Geometry check sheet. Reference: drawing and pictorial views, mm from the part's lowest x, y, z. Give positions to 0.01 mm unless a question says otherwise; leave off trailing zeros. Order: outer loops, then holes, each group sorted by start corner. A loop starts at its lowest first (then second) coordinate and runs counter-clockwise, first axis right, second up.
Item 1: Sectioned sample at D-D on y = 6.5. Record the boundary of the cut face in (x, z).
Item 2: Gauge pin test, flat ends, axial feed: P1, Ø3, axis at x = 7, y = 37.5, coming from the -Z side; P2, Ø10, axis at x = 8, z = 14, coming from the -Y side. Record the tip position at first contact, or that the pin passes through.
Item 3: Release check for a two-part mould opening along X. For the marked faces 1, 2 and 3 record: released by +X, released by -X, zero draft, split by the parting line, or undercut.
Item 4: Sectioned sample at B-B on z = 16. Record the boundary of the cut face in (x, y).
Item 5: Sectioned sample at C-C on z = 5.5. Record the boundary of the cut face in (x, y), and give its area (3 significant figures).
Item 6: Sectioned sample at A-A on x = 32.5. Record the boundary of the cut face in (y, z).
Item 7: Material ranges on line 1 along Y through (x, z) = (32.5, 6.75); line 2 along Y through (x, z) = (34.5, 14.5); line 3 along X through (y, z) = (38, 28), recorded low to high.
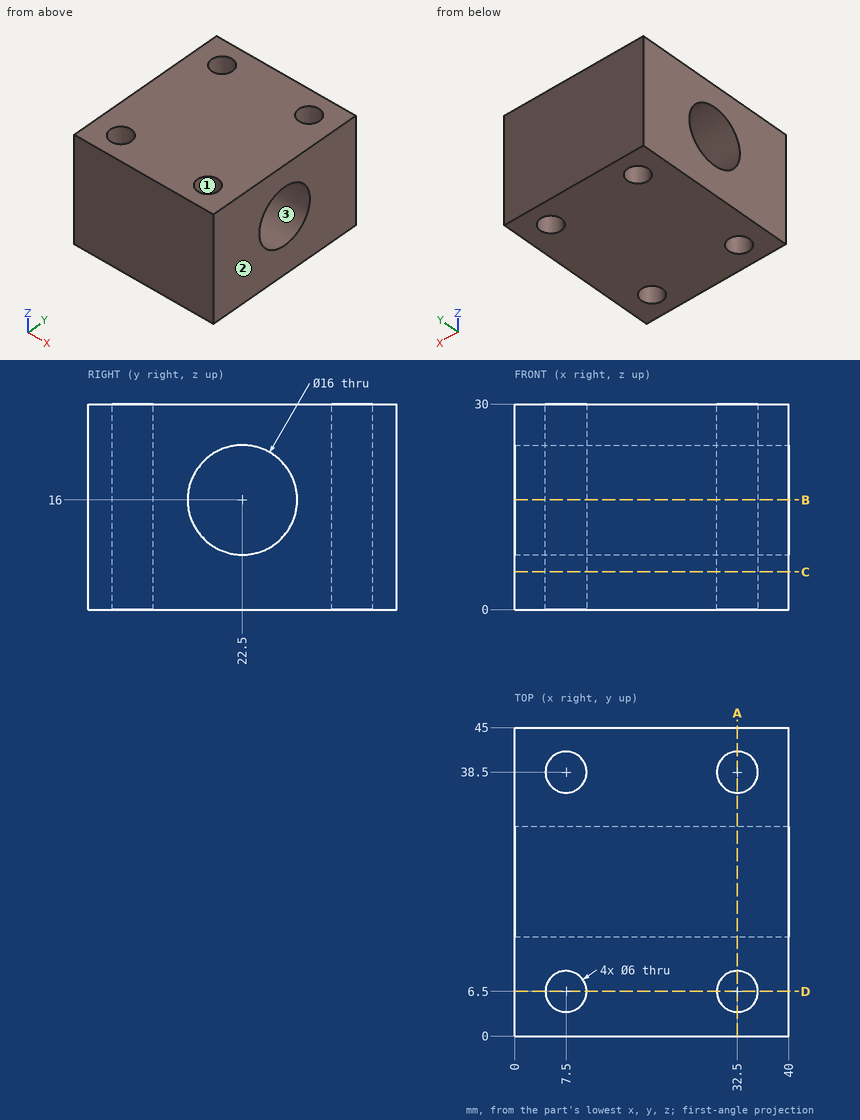
Report:
1. outline: (0, 0) - (4.5, 0) - (4.5, 30) - (0, 30) - close; (10.5, 0) - (29.5, 0) - (29.5, 30) - (10.5, 30) - close; (35.5, 0) - (40, 0) - (40, 30) - (35.5, 30) - close
2. P1: passes through
2. P2: stops at y = 0
3. face 1: undercut
3. face 2: released by +X
3. face 3: zero draft
4. outline: (0, 0) - (40, 0) - (40, 14.5) - (0, 14.5) - close; (0, 30.5) - (40, 30.5) - (40, 45) - (0, 45) - close; hole circle Ø6 at (7.5, 6.5); hole circle Ø6 at (7.5, 38.5); hole circle Ø6 at (32.5, 6.5); hole circle Ø6 at (32.5, 38.5)
5. outline: (0, 0) - (40, 0) - (40, 45) - (0, 45) - close; hole circle Ø6 at (7.5, 6.5); hole circle Ø6 at (7.5, 38.5); hole circle Ø6 at (32.5, 6.5); hole circle Ø6 at (32.5, 38.5)
5. area: 1,690 mm2
6. outline: (0, 0) - (3.5, 0) - (3.5, 30) - (0, 30) - close; (9.5, 0) - (35.5, 0) - (35.5, 30) - (9.5, 30) - close; (41.5, 0) - (45, 0) - (45, 30) - (41.5, 30) - close; hole circle Ø16 at (22.5, 16)
7. line 1: y = 0 to 3.5, 9.5 to 35.5, 41.5 to 45
7. line 2: y = 0 to 4.26, 8.74 to 14.64, 30.36 to 36.26, 40.74 to 45
7. line 3: x = 0 to 4.54, 10.46 to 29.54, 35.46 to 40
